```python
from build123d import *

# Parameters (mm, degrees)
BOX001_W               = 10
BOX001_H               = 2
BOX001_DEPTH           = 2
BOX001_PLACEMENT_ANGLE = 340
BOX_W                  = 10
BOX_H                  = 2
BOX_DEPTH              = 2
BOX_PLACEMENT_ANGLE    = 20


with BuildPart() as cube001:
    # Box001 → Box001 (new body)
    with BuildSketch(Plane.XY):
        with Locations((5, 1)):
            Rectangle(BOX001_W, BOX001_H)
    extrude(amount=BOX001_DEPTH)


with BuildPart() as cube001_1:
    # Box001 placement: moved
    add(cube001.part.moved(Location((-0.040483, 1.770408, 0))).rotate(Axis((-0.040483, 1.770408, 0), (0, 0, 1)), BOX001_PLACEMENT_ANGLE))


with BuildPart() as fusion:
    # Box → Box (new body)
    with BuildSketch(Plane.XY):
        with Locations((5, 1)):
            Rectangle(BOX_W, BOX_H)
    extrude(amount=BOX_DEPTH)


with BuildPart() as fusion_1:
    # Box placement: moved
    add(fusion.part.moved(Location((0.643557, -1.649793, 0))).rotate(Axis((0.643557, -1.649793, 0), (0, 0, 1)), BOX_PLACEMENT_ANGLE))

    # Fusion: union Cube001
    add(cube001_1.part)


solid = fusion_1.part
```
Geometry: final body of the model. Coordinates: model frame, mm. A direction names the side the tool comes from. Coordinates: 2 decimals unless noted, no trailing zeros. Order: outer loops, then holes, each group sorted by start corner. A loop starts at its lowest first (then second) coordinate and runs counter-clockwise, first axis right, second up. Notation, with made-up numbers: (25.5, 53) -> (50.5, 53) arc R24 cw to (50.5, 84) -> close; hole circle Ø9 at (20, -4). An arc over 180 degrees is marked (long way). Write item = value, one per line.
(1) Cut plane A-A on y = -1.05. Return loops of the section in (x, z).
Solved:
outline = (0.43, 0) -> (2.29, 0) -> (2.29, 2) -> (0.43, 2) -> close; (7.71, 0) -> (9.57, 0) -> (9.57, 2) -> (7.71, 2) -> close
(2) Line query: line 1 (Y direction, x = 1.5, z = 0.5); line 2 (Y direction, x = 9, z = 1.55); line 3 (Y direction, x = 5.75, z = 1). Output: solid intervals per line, ascending.
Solved:
line_1 = -1.34 to 0.79, 1.21 to 3.34
line_2 = -1.52 to 0.61, 1.39 to 3.52
line_3 = -0.34 to 2.34
(3) Cut plane C-C on x = 8.5. Return loops of the section in (y, z).
Solved:
outline = (-1.34, 0) -> (0.79, 0) -> (0.79, 2) -> (-1.34, 2) -> close; (1.21, 0) -> (3.34, 0) -> (3.34, 2) -> (1.21, 2) -> close
(4) Cut plane D-D on y = 1.2. Return loops of the section in (x, z).
Solved:
outline = (1.53, 0) -> (8.47, 0) -> (8.47, 2) -> (1.53, 2) -> close
(5) Cut plane B-B on z = 1.75. Return loops of the section in (x, y).
Solved:
outline = (-0.04, 0.23) -> (0.64, -1.65) -> (5, -0.06) -> (9.36, -1.65) -> (10.04, 0.23) -> (7.92, 1) -> (10.04, 1.77) -> (9.36, 3.65) -> (5, 2.06) -> (0.64, 3.65) -> (-0.04, 1.77) -> (2.08, 1) -> close
(6) Access query for faces 4 (the flat face through (7.148, -0.846, 0.986)), 5 (the flat face through (1, 1.39, 0.99)), 6 (the flat face through (8.97, 1.38, 0.99)). Directions: +Z, -Z, +X, -X, +Y, -Y. A direction counts if a zero-diameter tool reaches every point of the face in a straight line with its end or side. Return the directions, or none.
Solved:
face_4 = +Z, -Z, -Y
face_5 = +Z, -Z, -X
face_6 = +Z, -Z, +X
(7) Pull-direction query (Y, two-part tool) for faces 1 (the flat face through (7.148, 2.846, 0.986)), 2 (the flat face through (5, 1, 0)), 3 (the flat face through (8.97, 0.62, 0.99)); classes: pulls with the +Y half, pulls with the -Y half, needs draft (parallel to the pull), parting line crosses it, or undercut.
Solved:
face_1 = pulls with the +Y half
face_2 = needs draft
face_3 = undercut
